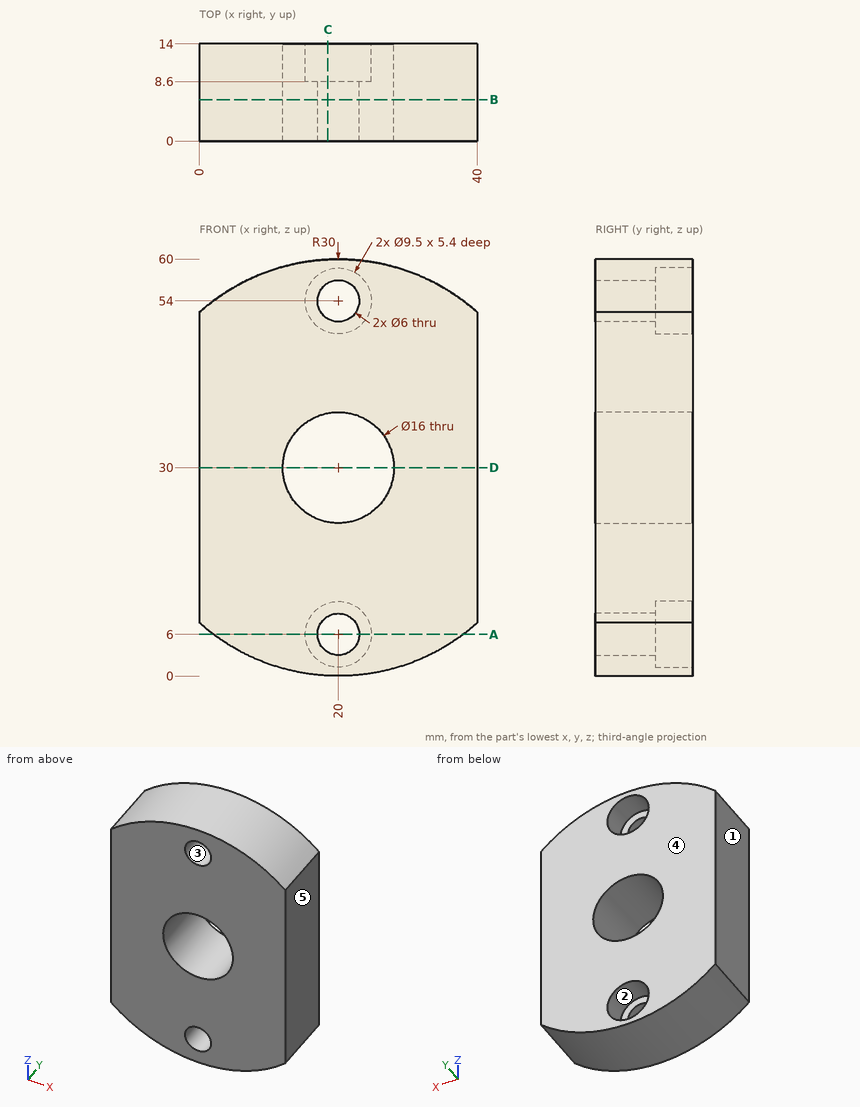
Geometry: see drawing. Coordinates: mm, zero at the bounding-box minimum. A direction names the side the tool comes from. Round coordinates to 2 decimals unless told otherwise and drop trailing zeros. Loops run counter-clockwise (first coordinate to the right, second up) from the corner with the lowest first, then second, coordinate; pieces in that order, holes last. Notation, with made-up numbers: M 82.25,62 L 101.25,62 A18 cw 101.25,66 Z; hole C -15,4 d4. An arc over 180 degrees is marked long. Use a Markdown table: item, result. Add a question column.
1. Section query B-B on y = 6. Return the cut outline in (x, z).
2. Section query C-C on x = 18.5. Return the cut outline in (y, z), then the cut area to 3 significant figures.
3. Reachability of the marked faces 1 and 2 from +Z, -Z, +X, -X, +Y, -Y: full face, straight path, thin tool, end or side. Return the list, or none.
4. Line query: line 1 (Z direction, x = 17.5, y = 13.25); line 2 (Z direction, x = 16.5, y = 10.75); line 3 (X direction, y = 8.5, z = 30). Output: solid intervals per line, ascending.
5. Mould query, pull axis X, two halves, no side actions, for the marked faces 3, 4 and 5. Classes: pulls with the +X half, pulls with the -X half, needs draft (parallel to the pull), parting line crosses it, or undercut.
6. Section query A-A on z = 6. Return the cut outline in (x, y).
7. Contact query for flat-ended pins moving along their axis: P1, Ø4, axis at x = 9.5, y = 8, coming from the -Z side; P2, Ø8.5, axis at x = 20, z = 54, coming from the +Y side; P3, Ø1.5, axis at x = 22, y = 9.5, coming from the +Z side. Output: stop coordinate, or through.
8. Section query D-D on z = 30. Return the cut outline in (x, y).
Reported:
| question | item | result |
|---|---|---|
| 1 | outline | M 0,7.64 A30 ccw 40,7.64 L 40,52.36 A30 ccw 0,52.36 Z; hole C 20,30 d16; hole C 20,6 d6; hole C 20,54 d6 |
| 2 | outline | M 0,0.04 L 14,0.04 L 14,1.49 L 8.6,1.49 L 8.6,3.4 L 0,3.4 Z; M 0,8.6 L 8.6,8.6 L 8.6,10.51 L 14,10.51 L 14,22.14 L 0,22.14 Z; M 0,37.86 L 14,37.86 L 14,49.49 L 8.6,49.49 L 8.6,51.4 L 0,51.4 Z; M 0,56.6 L 8.6,56.6 L 8.6,58.51 L 14,58.51 L 14,59.96 L 0,59.96 Z |
| 2 | area | 432 mm² |
| 3 | face 1 | +Z, -Z, -X, +Y, -Y |
| 3 | face 2 | +Y |
| 4 | line 1 | z = 0.1 to 1.96, 10.04 to 22.4, 37.6 to 49.96, 58.04 to 59.9 |
| 4 | line 2 | z = 0.2 to 2.79, 9.21 to 22.81, 37.19 to 50.79, 57.21 to 59.8 |
| 4 | line 3 | x = 0 to 12, 28 to 40 |
| 5 | face 3 | undercut |
| 5 | face 4 | needs draft |
| 5 | face 5 | pulls with the +X half |
| 6 | outline | M 2,0 L 17,0 L 17,8.6 L 15.25,8.6 L 15.25,14 L 2,14 Z; M 23,0 L 38,0 L 38,14 L 24.75,14 L 24.75,8.6 L 23,8.6 Z |
| 7 | P1 | stops at z = 1.23 |
| 7 | P2 | stops at y = 8.6 |
| 7 | P3 | stops at z = 59.97 |
| 8 | outline | M 0,0 L 12,0 L 12,14 L 0,14 Z; M 28,0 L 40,0 L 40,14 L 28,14 Z |
